Here's the drawing with two shaded views (mm, measured from the low corner). I have some questions. A direction names the side the tool comes from. Coordinates: 2 decimals unless noted, no trailing zeros. Order: outer loops, then holes, each group sorted by start corner. A loop starts at its lowest first (then second) coordinate and runs counter-clockwise, first axis right, second up. Notation, with made-up numbers: (-36.75, 45) -> (4.25, 45) arc R30 ccw to (4.25, 77) -> close; hole circle Ø4 at (-2, -26.5). An arc over 180 degrees is marked (long way). Answer as a JSON object with one key per item and string values. Group by question number.
(1) I want a section at D-D, the plane z = 21.25. List the corners of the cut face in (x, y) for me, plus the area to 3 significant figures.
(2) I want a section at C-C, the plane y = 2.55. List the corners of the cut face in (x, z) for me.
(3) I need wall thicknesses on line 1 (Z direction, x = 4.5, y = 3.15); line 2 (Z direction, x = 3, y = 2.75); line 3 (Z direction, x = 4.5, y = 1). Which ranges of each line are inside material? Lowest first, please.
(4) If we mould it in two halves opening along Z, with no side actions, what happens to the marked faces 1, 2, 3 and 4? For each: pulls with the +Z half, pulls with the -Z half, needs draft (parallel to the pull), parting line crosses it, or undercut.
(5) For pin 1 (1.5 mm diameter, centred on x = 1, y = 2, fed in from -Z), with a flat end and sliding along its axis, tell me the tip position at first contact or that it passes through.
(6) I want a section at A-A, the plane x = 4.5. List the corners of the cut face in (y, z) for me.
(7) Which directions (+Z, -Z, +X, -X, +Y, -Y) give clear straight access to the entire face, cutting with the end or side of a thin tool? Please do the marked faces 5 and 6.
(8) I want a section at B-B, the plane z = 5. List the corners of the cut face in (x, y) for me.
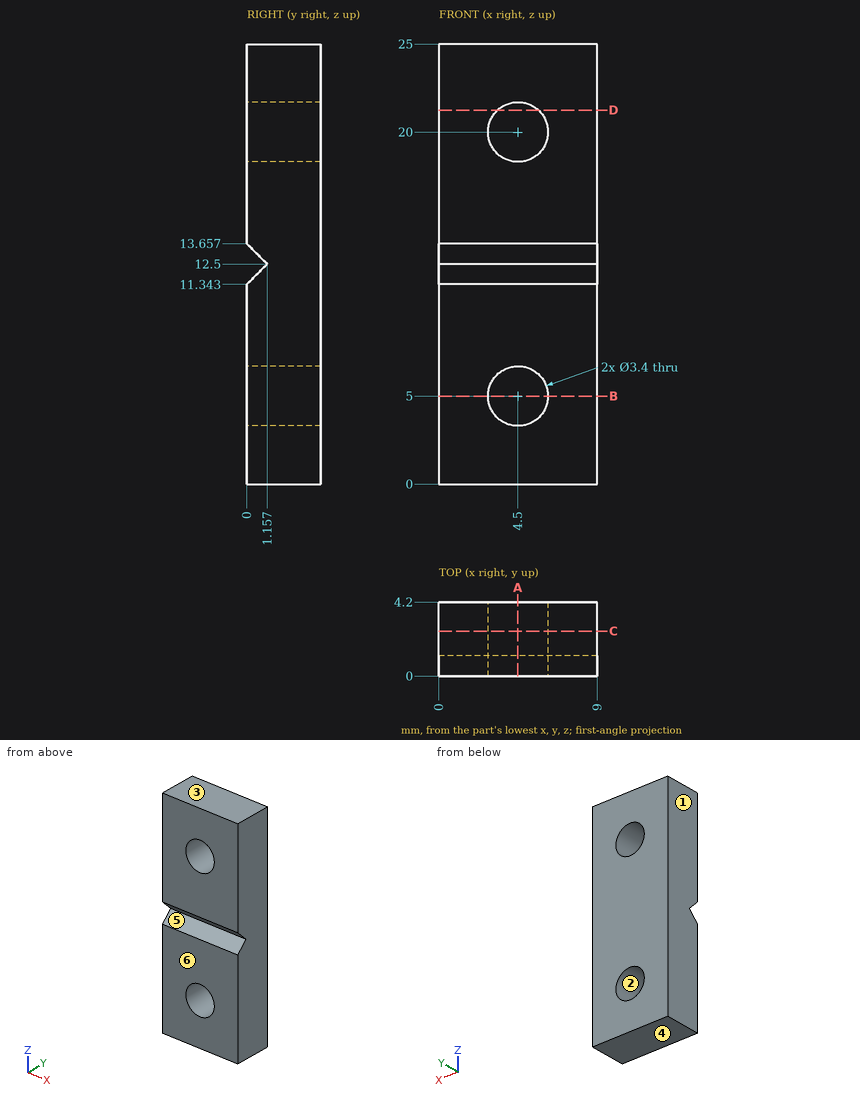
Computed values:
{
 "1": {"outline": "(0, 0) -> (3.35, 0) -> (3.35, 4.2) -> (0, 4.2) -> close; (5.65, 0) -> (9, 0) -> (9, 4.2) -> (5.65, 4.2) -> close", "area": "28.1 mm2"},
 "2": {"outline": "(0, 0) -> (9, 0) -> (9, 25) -> (0, 25) -> close; hole circle Ø3.4 at (4.5, 5); hole circle Ø3.4 at (4.5, 20)"},
 "3": {"line 1": "z = 0 to 3.3, 6.7 to 18.3, 21.7 to 25", "line 2": "z = 0 to 4.2, 5.8 to 19.2, 20.8 to 25", "line 3": "z = 0 to 3.3, 6.7 to 12.34, 12.66 to 18.3, 21.7 to 25"},
 "4": {"face 1": "needs draft", "face 2": "undercut", "face 3": "pulls with the +Z half", "face 4": "pulls with the -Z half"},
 "5": {"pin 1": "stops at z = 0"},
 "6": {"outline": "(0, 0) -> (4.2, 0) -> (4.2, 3.3) -> (0, 3.3) -> close; (0, 6.7) -> (4.2, 6.7) -> (4.2, 18.3) -> (0, 18.3) -> (0, 13.66) -> (1.16, 12.5) -> (0, 11.34) -> close; (0, 21.7) -> (4.2, 21.7) -> (4.2, 25) -> (0, 25) -> close"},
 "7": {"face 5": "+X, -X, -Y", "face 6": "+Z, -Z, +X, -X, -Y"},
 "8": {"outline": "(0, 0) -> (2.8, 0) -> (2.8, 4.2) -> (0, 4.2) -> close; (6.2, 0) -> (9, 0) -> (9, 4.2) -> (6.2, 4.2) -> close"}
}
